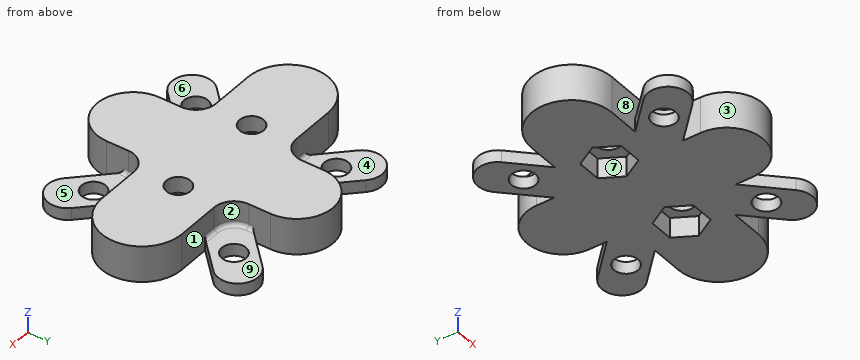
```python
from build123d import *

# Parameters (mm, degrees)
SKETCH1_R           = 3
BOSS_EXTRUDE2_DEPTH = 9
BOSS_EXTRUDE3_DEPTH = 9
CUT_EXTRUDE4_DEPTH  = 5
CUT_EXTRUDE5_START  = -6
SKETCH4_R           = 3
CUT_EXTRUDE5_DEPTH  = 6
FILLET1_R           = 5
FILLET2_R           = 1


with BuildPart() as part:
    # Sketch1 → Boss-Extrude2 (new body)
    # profile 1 of 3: a face of its own
    with BuildSketch(Plane.XY):
        with BuildLine():
            Line((17.67766953, -24.748737342), (-24.748737342, 17.67766953))
            ThreePointArc((-24.748737342, 17.67766953), (-24.748737342, 24.748737342), (-17.67766953, 24.748737342))
            Line((-17.67766953, 24.748737342), (24.748737342, -17.67766953))
            ThreePointArc((24.748737342, -17.67766953), (24.748737342, -24.748737342), (17.67766953, -24.748737342))
        make_face()
        with Locations((-17.5, 17.5)):
            Circle(SKETCH1_R, mode=Mode.SUBTRACT)
        with Locations((17.5, -17.5)):
            Circle(SKETCH1_R, mode=Mode.SUBTRACT)
    # profile 2 of 3: a face of its own
    with BuildSketch(Plane.XY):
        with BuildLine():
            Line((-24.748737342, -17.67766953), (17.67766953, 24.748737342))
            ThreePointArc((17.67766953, 24.748737342), (24.748737342, 24.748737342), (24.748737342, 17.67766953))
            Line((24.748737342, 17.67766953), (-17.67766953, -24.748737342))
            ThreePointArc((-17.67766953, -24.748737342), (-24.748737342, -24.748737342), (-24.748737342, -17.67766953))
        make_face()
        with Locations((17.5, 17.5)):
            Circle(SKETCH1_R, mode=Mode.SUBTRACT)
        with Locations((-17.5, -17.5)):
            Circle(SKETCH1_R, mode=Mode.SUBTRACT)
    # profile 3 of 3: a face of its own
    with BuildSketch(Plane.XY):
        with BuildLine():
            Line((-25, 10), (25, 10))
            ThreePointArc((25, 10), (35, 0), (25, -10))
            Line((25, -10), (-25, -10))
            ThreePointArc((-25, -10), (-35, 0), (-25, 10))
        make_face()
        with Locations((12.5, 0)):
            Circle(SKETCH1_R, mode=Mode.SUBTRACT)
        with Locations((-12.5, 0)):
            Circle(SKETCH1_R, mode=Mode.SUBTRACT)
    extrude(amount=BOSS_EXTRUDE2_DEPTH)

    # Sketch5 → Boss-Extrude3 (add)
    with BuildSketch(Plane.XY.offset(9)):
        with BuildLine():
            Line((9, 20.422973397), (9, -20.422973397))
            ThreePointArc((9, -20.422973397), (0, -29.422973397), (-9, -20.422973397))
            Line((-9, -20.422973397), (-9, 20.422973397))
            ThreePointArc((-9, 20.422973397), (0, 29.422973397), (9, 20.422973397))
        make_face()
    extrude(amount=-BOSS_EXTRUDE3_DEPTH)

    # Sketch6 → Cut-Extrude4 (cut)
    with BuildSketch(Plane(origin=(0, 0, 0), x_dir=(-1, 0, 0), z_dir=(0, 0, -1))):
        Polygon((-6.611027254, 0), (-9.555513627, 5.1), (-15.444486373, 5.1), (-18.388972746, 0), (-15.444486373, -5.1), (-9.555513627, -5.1), align=None)
        Polygon((17.886314115, 0.120263137), (14.941827742, 5.220263137), (9.052854996, 5.220263137), (6.108368623, 0.120263137), (9.052854996, -4.979736863), (14.941827742, -4.979736863), align=None)
    extrude(amount=-CUT_EXTRUDE4_DEPTH, mode=Mode.SUBTRACT)

    # Sketch4 → Cut-Extrude5 (cut)
    # profile 1 of 8: a face of its own
    with BuildSketch(Plane.XY.offset(9).offset(CUT_EXTRUDE5_START)):
        with BuildLine():
            Line((-9, 26.683350041), (-29.894469541, 26.683350041))
            Line((-29.894469541, 26.683350041), (-29.894469541, 10))
            Line((-29.894469541, 10), (-25, 10))
            Line((-25, 10), (-17.071067812, 10))
            Line((-17.071067812, 10), (-24.748737342, 17.67766953))
            ThreePointArc((-24.748737342, 17.67766953), (-24.748737342, 24.748737342), (-17.67766953, 24.748737342))
            Line((-17.67766953, 24.748737342), (-9, 16.071067812))
            Line((-9, 16.071067812), (-9, 20.422973397))
            Line((-9, 20.422973397), (-9, 26.683350041))
        make_face()
    # profile 2 of 8: a face of its own
    with BuildSketch(Plane.XY.offset(9).offset(CUT_EXTRUDE5_START)):
        with BuildLine():
            Line((-9, 10), (-9, 16.071067812))
            Line((-9, 16.071067812), (-17.67766953, 24.748737342))
            ThreePointArc((-17.67766953, 24.748737342), (-24.748737342, 24.748737342), (-24.748737342, 17.67766953))
            Line((-24.748737342, 17.67766953), (-17.071067812, 10))
            Line((-17.071067812, 10), (-9, 10))
        make_face()
        with Locations((-17.5, 17.5)):
            Circle(SKETCH4_R, mode=Mode.SUBTRACT)
    # profile 3 of 8: a face of its own
    with BuildSketch(Plane.XY.offset(9).offset(CUT_EXTRUDE5_START)):
        with BuildLine():
            Line((25, 10), (29.894469541, 10))
            Line((29.894469541, 10), (29.894469541, 26.683350041))
            Line((29.894469541, 26.683350041), (9, 26.683350041))
            Line((9, 26.683350041), (9, 20.422973397))
            Line((9, 20.422973397), (9, 16.071067812))
            Line((9, 16.071067812), (17.67766953, 24.748737342))
            ThreePointArc((17.67766953, 24.748737342), (24.748737342, 24.748737342), (24.748737342, 17.67766953))
            Line((24.748737342, 17.67766953), (17.071067812, 10))
            Line((17.071067812, 10), (25, 10))
        make_face()
    # profile 4 of 8: a face of its own
    with BuildSketch(Plane.XY.offset(9).offset(CUT_EXTRUDE5_START)):
        with BuildLine():
            Line((9, 10), (17.071067812, 10))
            Line((17.071067812, 10), (24.748737342, 17.67766953))
            ThreePointArc((24.748737342, 17.67766953), (24.748737342, 24.748737342), (17.67766953, 24.748737342))
            Line((17.67766953, 24.748737342), (9, 16.071067812))
            Line((9, 16.071067812), (9, 10))
        make_face()
        with Locations((17.5, 17.5)):
            Circle(SKETCH4_R, mode=Mode.SUBTRACT)
    # profile 5 of 8: a face of its own
    with BuildSketch(Plane.XY.offset(9).offset(CUT_EXTRUDE5_START)):
        with BuildLine():
            Line((9, -26.683350041), (29.894469541, -26.683350041))
            Line((29.894469541, -26.683350041), (29.894469541, -10))
            Line((29.894469541, -10), (25, -10))
            Line((25, -10), (17.071067812, -10))
            Line((17.071067812, -10), (24.748737342, -17.67766953))
            ThreePointArc((24.748737342, -17.67766953), (24.748737342, -24.748737342), (17.67766953, -24.748737342))
            Line((17.67766953, -24.748737342), (9, -16.071067812))
            Line((9, -16.071067812), (9, -20.422973397))
            Line((9, -20.422973397), (9, -26.683350041))
        make_face()
    # profile 6 of 8: a face of its own
    with BuildSketch(Plane.XY.offset(9).offset(CUT_EXTRUDE5_START)):
        with BuildLine():
            Line((24.748737342, -17.67766953), (17.071067812, -10))
            Line((17.071067812, -10), (9, -10))
            Line((9, -10), (9, -16.071067812))
            Line((9, -16.071067812), (17.67766953, -24.748737342))
            ThreePointArc((17.67766953, -24.748737342), (24.748737342, -24.748737342), (24.748737342, -17.67766953))
        make_face()
        with Locations((17.5, -17.5)):
            Circle(SKETCH4_R, mode=Mode.SUBTRACT)
    # profile 7 of 8: a face of its own
    with BuildSketch(Plane.XY.offset(9).offset(CUT_EXTRUDE5_START)):
        with BuildLine():
            Line((-9, -10), (-17.071067812, -10))
            Line((-17.071067812, -10), (-24.748737342, -17.67766953))
            ThreePointArc((-24.748737342, -17.67766953), (-24.748737342, -24.748737342), (-17.67766953, -24.748737342))
            Line((-17.67766953, -24.748737342), (-9, -16.071067812))
            Line((-9, -16.071067812), (-9, -10))
        make_face()
        with Locations((-17.5, -17.5)):
            Circle(SKETCH4_R, mode=Mode.SUBTRACT)
    # profile 8 of 8: a face of its own
    with BuildSketch(Plane.XY.offset(9).offset(CUT_EXTRUDE5_START)):
        with BuildLine():
            Line((-25, -10), (-29.894469541, -10))
            Line((-29.894469541, -10), (-29.894469541, -26.683350041))
            Line((-29.894469541, -26.683350041), (-9, -26.683350041))
            Line((-9, -26.683350041), (-9, -20.422973397))
            Line((-9, -20.422973397), (-9, -16.071067812))
            Line((-9, -16.071067812), (-17.67766953, -24.748737342))
            ThreePointArc((-17.67766953, -24.748737342), (-24.748737342, -24.748737342), (-24.748737342, -17.67766953))
            Line((-24.748737342, -17.67766953), (-17.071067812, -10))
            Line((-17.071067812, -10), (-25, -10))
        make_face()
    extrude(amount=CUT_EXTRUDE5_DEPTH, mode=Mode.SUBTRACT)

    # Fillet1
    fillet1_edges = [part.edges().sort_by_distance(p)[0] for p in [
        (-9, -10, 6),
        (9, -10, 6),
        (9, 10, 6),
        (-9, 10, 6),
    ]]
    fillet(fillet1_edges, radius=FILLET1_R)

    # Fillet2
    fillet2_edges = [part.edges().sort_by_distance(p)[0] for p in [
        (-9, -15.535533906, 3),
        (-15.535533906, -10, 3),
        (15.535533906, -10, 3),
        (9, -15.535533906, 3),
        (9, 15.535533906, 3),
        (15.535533906, 10, 3),
        (-15.535533906, 10, 3),
        (-9, 15.535533906, 3),
        (10.464466094, 11.464466094, 3),
        (-10.464466094, 11.464466094, 3),
        (-10.464466094, -11.464466094, 3),
        (10.464466094, -11.464466094, 3),
    ]]
    fillet(fillet2_edges, radius=FILLET2_R)


solid = part.part
```
CAD build for the part. Positions are in the model's coordinates, mm. Face numbers are marked on the shaded views. A direction names the side the tool comes from. Round coordinates to 2 decimals unless told otherwise and drop trailing zeros. Loops run counter-clockwise (first coordinate to the right, second up) from the corner with the lowest first, then second, coordinate; pieces in that order, holes last. Notation, with made-up numbers: M 44.25,19 L 92.25,19 A16 ccw 92.25,29 Z; hole C 31,28.5 d11. An arc over 180 degrees is marked long. Return JSON: item names as keys, results as strings. Group by question number.
(1) Saw through at B-B, the plane y = -2. List the corners of the cut face in (x, z).
(2) Saw through at A-A, the plane z = 8.25. List the corners of the cut face in (x, y), and give its area (3 significant figures).
(3) Saw through at C-C, the plane x = 23. List the corners of the cut face in (y, z), and give its area (3 significant figures).
(4) Drop flat-ended pins along their axis: P1, Ø2.5, axis at x = -12, z = 3, coming from the -Y side; P2, Ø5, axis at y = 14.5, z = 6.5, coming from the +X side; P3, Ø4.5, axis at x = 22, z = 4, coming from the -Y side. Give the stop position or say it passes through.
(5) Wall check: probe 1 along X at (y, z) = (0, 7.75); probe 2 along X at (y, z) = (2, 8.25); probe 3 along Y at (x, z) = (-17.5, 2.25). Give the ranges that are in metal, low to high. Write a range as [from, to].
(6) Saw through at D-D, the plane y = -22.5. List the corners of the cut face in (x, z).
(7) Tool access for the marked faces 5, 6, 7, 8 and 9: list every direction of +Z, -Z, +X, -X, +Y, -Y with a clear straight run to the whole face (end or side of a thin tool).
(8) Mould opens along Y. For the marked faces 1, 2, 3 and 4 say: +Y half, -Y half, draft (parallel to the pull), parting line (faces both ways), or undercut.
Answer list:
{
 "1": {"outline": "M -34.8,0 L -16.66,0 L -16.66,5 L -14.74,5 L -14.74,9 L -34.8,9 Z; M -10.26,5 L -7.33,5 L -7.33,0 L 7.77,0 L 7.77,5 L 10.26,5 L 10.26,9 L -10.26,9 Z; M 14.74,5 L 17.23,5 L 17.23,0 L 34.8,0 L 34.8,9 L 14.74,9 Z"},
 "2": {"outline": "M -25,-10 L -14,-10 A5 cw -9,-15 L -9,-20.42 A9 ccw 9,-20.42 L 9,-15 A5 cw 14,-10 L 25,-10 A10 ccw 25,10 L 14,10 A5 cw 9,15 L 9,20.42 A9 ccw -9,20.42 L -9,15 A5 cw -14,10 L -25,10 A10 ccw Z; hole C -12.5,0 d6; hole C 12.5,0 d6", "area": "1,910 mm2"},
 "3": {"outline": "M -25.88,0 L -15.93,0 L -15.93,3 L -25.88,3 Z; M -10,0 L 10,0 L 10,9 L -10,9 Z; M 15.93,0 L 25.88,0 L 25.88,3 L 15.93,3 Z", "area": "240 mm2"},
 "4": {"P1": "y = -20.32", "P2": "x = 10", "P3": "y = -26.21"},
 "5": {"probe 1": "[-35, -15.5], [-9.5, 9.5], [15.5, 35]", "probe 2": "[-34.8, -14.74], [-10.26, 10.26], [14.74, 34.8]", "probe 3": "[-24.57, -20.5], [-14.5, -10.43], [-10, -0.55], [0.79, 10], [10.43, 14.5], [20.5, 24.57]"},
 "6": {"outline": "M -26.04,0 L -15.43,0 L -15.43,3 L -26.04,3 Z; M -8.76,0 L 8.76,0 L 8.76,9 L -8.76,9 Z; M 15.43,0 L 26.04,0 L 26.04,3 L 15.43,3 Z"},
 "7": {"face 5": "+Z, +X, -Y", "face 6": "+Z, -X, -Y", "face 7": "-Z", "face 8": "+Z, -X", "face 9": "+Z, +X, +Y"},
 "8": {"face 1": "undercut", "face 2": "+Y half", "face 3": "-Y half", "face 4": "draft"}
}
